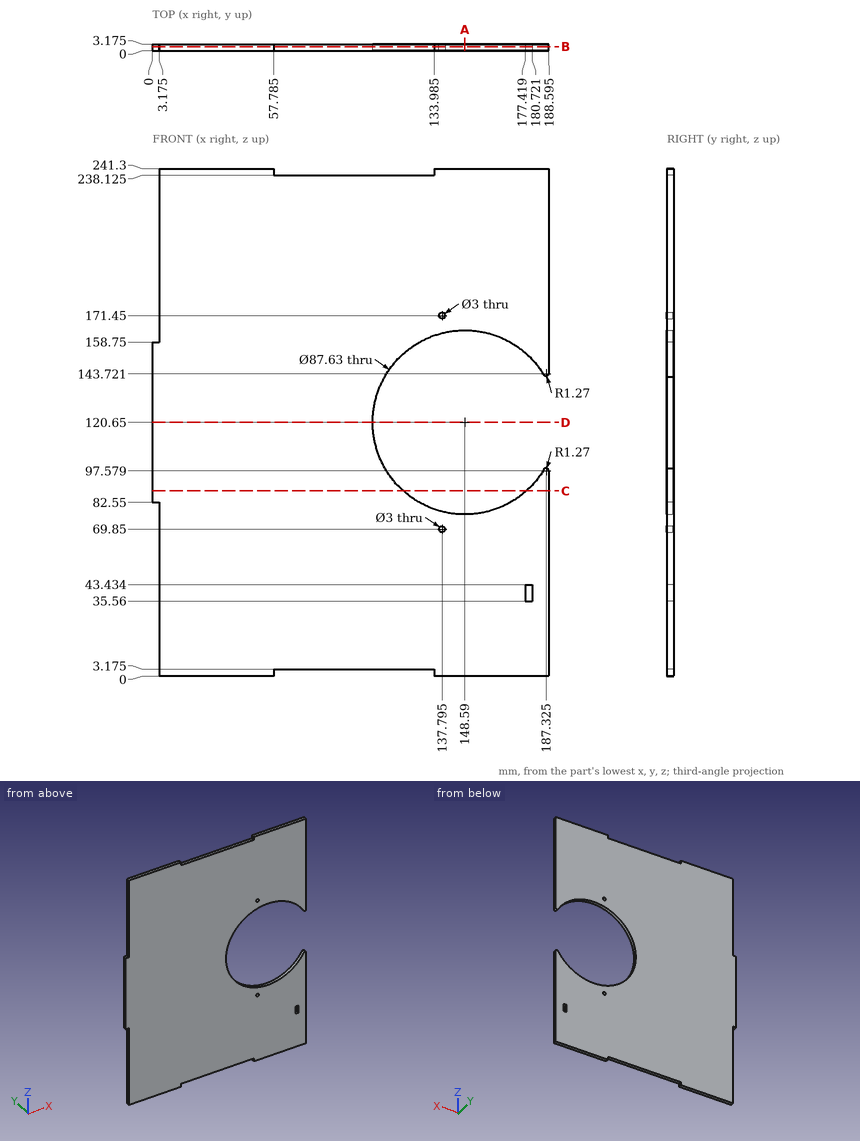
Print and shaded views of the part. All mm, measured from the part's lowest x, y and z. Round coordinates to 2 decimals unless told otherwise and drop trailing zeros. Loops run counter-clockwise (first coordinate to the right, second up) from the corner with the lowest first, then second, coordinate; pieces in that order, holes last. Notation, with made-up numbers: M 57,67.25 L 66,67.25 A23 ccw 66,81.25 Z; hole C 81,-30.75 d6. An arc over 180 degrees is marked long. One line per question, with ' | ' between items.
1) Flat gauge pins, fed straight in: pin 1 (1.6 mm diameter, centred on x = 1.5, y = 1.5, fed in from +Z); pin 2 (1 mm diameter, centred on y = 1.5, z = 39, fed in from -X) (3 decimals); pin 3 (1 mm diameter, centred on x = 1, y = 1, fed in from -Z). Where does each tip first touch, or does it go through?
Solved:
pin 1: stops at z = 158.75 | pin 2: stops at x = 3.175 | pin 3: stops at z = 82.55
2) Band-saw the part on A-A (x = 148.59). Give the cut face in (y, z) (1 decimal).
Solved:
outline: M 0,0 L 3.2,0 L 3.2,76.8 L 0,76.8 Z; M 0,164.5 L 3.2,164.5 L 3.2,241.3 L 0,241.3 Z
3) Band-saw the part on C-C (z = 88). Give the cut face in (x, y) (1 decimal).
Solved:
outline: M 0,0 L 119.4,0 L 119.4,3.2 L 0,3.2 Z; M 177.8,0 L 188.6,0 L 188.6,3.2 L 177.8,3.2 Z
4) Band-saw the part on B-B (y = 1.9). Give the number of separate pieces and of enclosed holes in the cut face, then the cut area to 3 significant figures.
Solved:
separate pieces: 1 | enclosed holes: 3 | area: 38,500 mm²
5) Drill centre lines: line 1 along Z through (x, y) = (148.59, 2.25) (1 decimal); line 2 along X through (y, z) = (2, 150.5) (1 decimal); line 3 along Z through (x, y) = (127.5, 3) (1 decimal). Where is each one in solid material? Low to high.
Solved:
line 1: z = 0 to 76.8, 164.5 to 241.3 | line 2: x = 0 to 116.5, 180.7 to 188.6 | line 3: z = 3.2 to 82.2, 159.1 to 238.1
6) Band-saw the part on D-D (z = 120.65). Give the cut face in (x, y) (1 decimal).
Solved:
outline: M 0,0 L 104.8,0 L 104.8,3.2 L 0,3.2 Z
